Can you work these out from the drawing? Everything is in mm from the part's minimum corner. A direction names the side the tool comes from. Round coordinates to 2 decimals unless told otherwise and drop trailing zeros. Write each loop counter-clockwise with the first axis right and the second up, starting at its lowest first coordinate (ties: lowest second). Pieces come first, ordered by that corner, then holes. Notation, with made-up numbers: (3.25, 5.25) -> (46.25, 5.25) arc R27 ccw to (46.25, 37.25) -> close; hole circle Ø7 at (75.5, -3.5). An arc over 180 degrees is marked (long way). One line per question, with ' | ' between items. Start each with the question number.
1. For pin 1 Ø11.5 at (x, z) = (11, 62.5) entering from +Y; pin 2 Ø2.5 at (y, z) = (7.62, 7.45) entering from +X, each with a flat end and sliding along its axis, tell me the tip position at first contact or that it passes through.
2. Thinking about a two-plate mould opening in X: for the marked faces 3, 4 and 5, which applies, released by +X, released by -X, zero draft, split by the parting line, or undercut?
3. Imagine slicing it at B-B, the plane x = 16. List the corners of the cut face in (y, z) for me, and give its area (3 significant figures).
4. If I drill on line 1 along Z through (x, y) = (6, 7); line 2 along Z through (x, y) = (24.9, 7.62); line 3 along X through (y, z) = (5.5, 71.5), over which ranges is the centre line in solid material (lowest first)? Write a range as [from, to].
5. Imagine slicing it at A-A, the plane y = 10.25. List the corners of the cut face in (x, z) for me, and give its area (3 significant figures).
6. Imagine slicing it at C-C, the plane z = 58.5. List the corners of the cut face in (x, y) for me.
7. For the marked faces 1 and 2, which set-ups out of +Z, -Z, +X, -X, +Y, -Y let a thin tool reach every point of the face, with its end or its side?
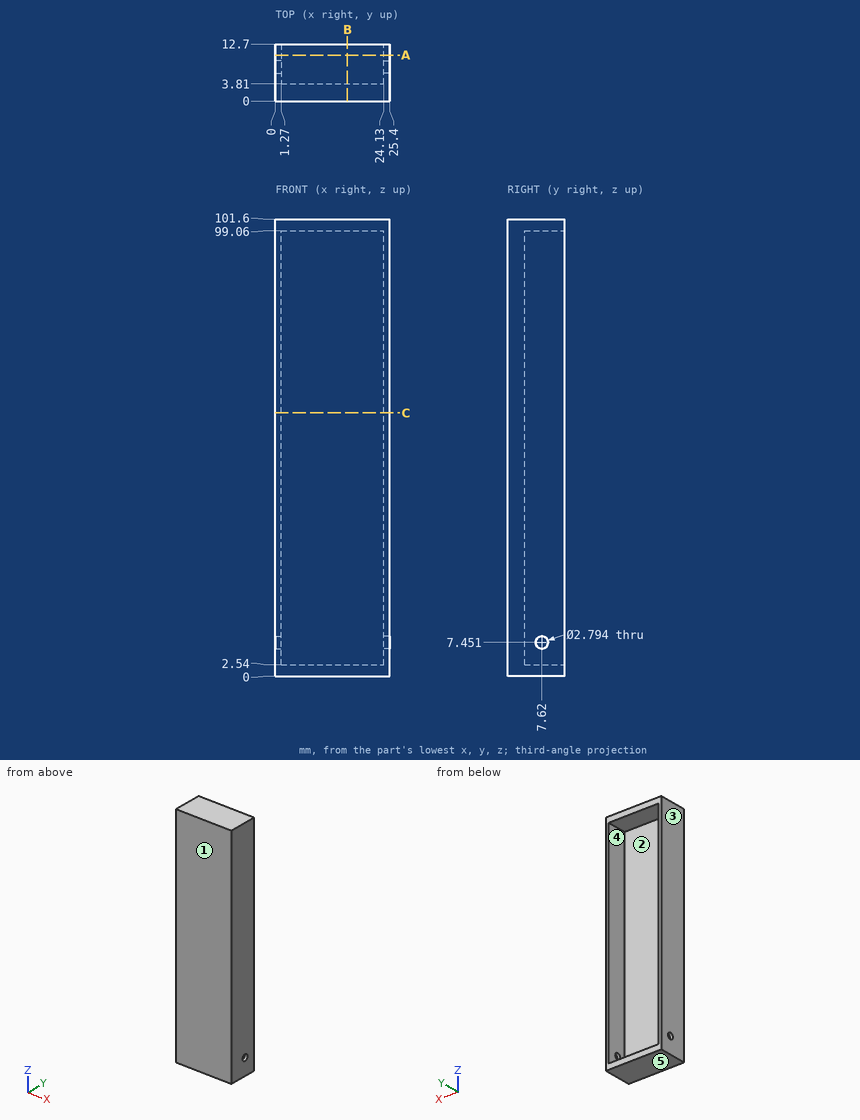
Geometry results:
1) pin 1: stops at y = 3.81 | pin 2: passes through
2) face 3: released by -X | face 4: undercut | face 5: zero draft
3) outline: (0, 0) -> (12.7, 0) -> (12.7, 2.54) -> (3.81, 2.54) -> (3.81, 99.06) -> (12.7, 99.06) -> (12.7, 101.6) -> (0, 101.6) -> close | area: 432 mm2
4) line 1: z = [0, 2.54], [99.06, 101.6] | line 2: z = [0, 6.05], [8.85, 101.6] | line 3: x = [0, 1.27], [24.13, 25.4]
5) outline: (0, 0) -> (25.4, 0) -> (25.4, 101.6) -> (0, 101.6) -> close; hole (1.27, 2.54) -> (24.13, 2.54) -> (24.13, 99.06) -> (1.27, 99.06) -> close | area: 374 mm2
6) outline: (0, 0) -> (25.4, 0) -> (25.4, 12.7) -> (24.13, 12.7) -> (24.13, 3.81) -> (1.27, 3.81) -> (1.27, 12.7) -> (0, 12.7) -> close
7) face 1: +Z, -Z, +X, -X, -Y | face 2: +Y
